```python
from build123d import *

# Parameters (mm, degrees)
SKETCH1_R           = 40
BOSS_EXTRUDE1_DEPTH = 2.54
SKETCH2_R           = 0.75
CUT_EXTRUDE1_DEPTH  = 10
SKETCH3_R           = 30.7
SKETCH3_R_2         = 26.7
BOSS_EXTRUDE2_DEPTH = 0.254


with BuildPart() as part:
    # Sketch1 → Boss-Extrude1 (new body)
    with BuildSketch(Plane(origin=(0, 0, 0), x_dir=(1, 0, 0), z_dir=(0, 1, 0))):
        Circle(SKETCH1_R)
    extrude(amount=BOSS_EXTRUDE1_DEPTH)

    # Sketch2 → Cut-Extrude1 (cut)
    with BuildSketch(Plane(origin=(0, 2.54, 0), x_dir=(1, 0, 0), z_dir=(0, 1, 0))):
        with Locations((0, 11)):
            Circle(SKETCH2_R)
        with Locations((9.526279442, -5.5)):
            Circle(SKETCH2_R)
        with Locations((-9.526279442, -5.5)):
            Circle(SKETCH2_R)
    extrude(amount=-CUT_EXTRUDE1_DEPTH, mode=Mode.SUBTRACT)

    # Sketch3 → Boss-Extrude2 (add)
    with BuildSketch(Plane.XZ):
        Circle(SKETCH3_R)
        Circle(SKETCH3_R_2, mode=Mode.SUBTRACT)
    extrude(amount=BOSS_EXTRUDE2_DEPTH)


solid = part.part
```
Input: part model. Units: mm. Frame: model coordinates. A direction names the side the tool comes from. Coordinates: 2 decimals unless noted, no trailing zeros. Loops run counter-clockwise (first coordinate to the right, second up) from the corner with the lowest first, then second, coordinate; pieces in that order, holes last.
Q1. Contact query for flat-ended pins moving along their axis: pin 1 (1.2 mm diameter, centred on x = -9.53, z = 5.5, fed in from +Y); pin 2 (1 mm diameter, centred on x = 21, y = 0.5, fed in from -Z); pin 3 (1.5 mm diameter, centred on x = 3, z = 4, fed in from -Y); pin 4 (1 mm diameter, centred on x = -8.5, y = 0, fed in from +Z). Output: stop coordinate, or through.
Results are:
pin 1: passes through
pin 2: stops at z = -34.35
pin 3: stops at y = 0
pin 4: stops at z = 39.19
Q2. Section C-C, the plane y = 1.5. Return the cut outline in (x, z).
Results are:
outline: circle Ø80 at (0, 0); hole circle Ø1.5 at (-9.53, 5.5); hole circle Ø1.5 at (0, -11); hole circle Ø1.5 at (9.53, 5.5)
Q3. Section A-A, the plane z = 0. Return the cut outline in (x, y), and give its area (3 significant figures).
Results are:
outline: (-40, 0) - (-30.7, 0) - (-30.7, -0.25) - (-26.7, -0.25) - (-26.7, 0) - (26.7, 0) - (26.7, -0.25) - (30.7, -0.25) - (30.7, 0) - (40, 0) - (40, 2.54) - (-40, 2.54) - close
area: 205 mm2
Q4. Section B-B, the plane x = -5.5. Return the cut outline in (y, z), and give its area (3 significant figures).
Results are:
outline: (-0.25, -30.2) - (0, -30.2) - (0, -39.62) - (2.54, -39.62) - (2.54, 39.62) - (0, 39.62) - (0, 30.2) - (-0.25, 30.2) - (-0.25, 26.13) - (0, 26.13) - (0, -26.13) - (-0.25, -26.13) - close
area: 203 mm2
Q5. Line query: line 1 along X through (y, z) = (1.65, -11); line 2 along Y through (x, z) = (-14.5, 29.5); line 3 along Z through (x, y) = (-9.5, 1.7). Output: solid intervals per line, ascending.
Results are:
line 1: x = -38.46 to -0.75, 0.75 to 38.46
line 2: y = 0 to 2.54
line 3: z = -38.86 to 4.75, 6.25 to 38.86
Q6. Set-up query: faces 1 (the flat face through (21, 0, 24)), 2 (the flat face through (-1, 2.54, -1)). Return all of +Z, -Z, +X, -X, +Y, -Y with unobstructed straight access to the full face (end or side cutting, diameter ignored); none if empty.
Results are:
face 1: -Y
face 2: +Z, -Z, +X, -X, +Y
